Geometry: final body of the model. Coordinates: model frame, mm. A direction names the side the tool comes from. Coordinates: 2 decimals unless noted, no trailing zeros. Loops run counter-clockwise (first coordinate to the right, second up) from the corner with the lowest first, then second, coordinate; pieces in that order, holes last. Notation, with made-up numbers: (41.25, 37) -> (98.25, 37) arc R18 cw to (98.25, 53) -> close; hole circle Ø4 at (-23, 83.25). An arc over 180 degrees is marked (long way). One line per item, written item: value. Start each with the question number.
Item 1: Ray query, probe 1 along Y at (x, z) = (6, 0); probe 2 along Y at (x, z) = (-4, 0); probe 3 along X at (y, z) = (-1.75, -0.25). Return the intervals inside material, ascending. Write a range as from..to.
Item 2: Contact query for flat-ended pins moving along their axis: pin 1 Ø1 at (x, y) = (-7.5, -1) entering from -Z; pin 2 Ø1.5 at (x, y) = (7, 0) entering from +Z; pin 3 Ø4 at (x, y) = (-7, -2.5) entering from +Z. Output: stop coordinate, or through.
Item 3: Section query A-A on y = 0. Return loops of the section in (x, z).
Item 4: Mould query, pull axis X, two halves, no side actions, for faces 1 (the cylindrical face through (5.07, -0.07, -1.5)), 2 (the flat face through (-10, 2, 2)), 3 (the cylindrical face through (-5.81, 0.38, 2.8)), 4 (the cylindrical face through (6.079, 0.845, 2.57)). Classes: +X half, -X half, draft (parallel to the pull), parting line (faces both ways), or undercut.
Item 5: Set-up query: faces 5 (the cylindrical face through (-5, 0, -2)), 6 (the cylindrical face through (-0.136, 3.905, -0.867)). Return all of +Z, -Z, +X, -X, +Y, -Y with unobstructed straight access to the full face (end or side cutting, diameter ignored); none if empty.
Item 6: Section query C-C on x = 5.25. Return loops of the section in (y, z).
Item 7: Section query B-B on z = 0. Return loops of the section in (x, y), then the cut area to 3 significant figures.
Item 8: Section query D-D on z = 3.25. Give the number of separate pieces and of enclosed holes in the cut face, then the cut area to 3 significant figures.
from build123d import *

# Parameters (mm, degrees)
ESQUISSE2_R             = 1.25
ENL_V_MAT_EXTRU_1_DEPTH = 5


with BuildPart() as part:
    # Esquisse1 → Révolution1 (revolve)
    with BuildSketch(Plane.XY, mode=Mode.PRIVATE) as r_volution1_sk:
        Polygon((-10, 3.7), (-10, 2), (0, 2), (0, 1.5), (10, 1.5), (10, 3.7), (9.7, 4), (-9.7, 4), align=None)
    revolve(r_volution1_sk.sketch.rotate(Axis((-9.079951531, 0, 0), (1, 0, 0)), 90), axis=Axis((-9.079951531, 0, 0), (1, 0, 0)))

    # Esquisse2 → Enlèv. mat.-Extru.1 (cut)
    with BuildSketch(Plane.XY.offset(6.1)):
        with Locations((-7, 0)):
            Circle(ESQUISSE2_R)
        with Locations((7, 0)):
            Circle(ESQUISSE2_R)
    extrude(amount=-ENL_V_MAT_EXTRU_1_DEPTH, mode=Mode.SUBTRACT)


solid = part.part
Reply:
1. probe 1: y = -4..-1.5, 1.5..4
1. probe 2: y = -4..-2, 2..4
1. probe 3: x = 0..10
2. pin 1: stops at z = -3.97
2. pin 2: stops at z = -1.3
2. pin 3: stops at z = 3.93
3. outline: (-10, -3.7) -> (-9.7, -4) -> (9.7, -4) -> (10, -3.7) -> (10, -1.5) -> (0, -1.5) -> (0, -2) -> (-10, -2) -> close; (-10, 2) -> (-8.25, 2) -> (-8.25, 4) -> (-9.7, 4) -> (-10, 3.7) -> close; (-5.75, 2) -> (0, 2) -> (0, 1.5) -> (5.75, 1.5) -> (5.75, 4) -> (-5.75, 4) -> close; (8.25, 1.5) -> (10, 1.5) -> (10, 3.7) -> (9.7, 4) -> (8.25, 4) -> close
4. face 1: draft
4. face 2: -X half
4. face 3: undercut
4. face 4: undercut
5. face 5: -X
5. face 6: +X, -X
6. outline: circle Ø8 at (0, 0); hole circle Ø3 at (0, 0)
7. outline: (-10, -3.7) -> (-9.7, -4) -> (9.7, -4) -> (10, -3.7) -> (10, -1.5) -> (0, -1.5) -> (0, -2) -> (-10, -2) -> close; (-10, 2) -> (0, 2) -> (0, 1.5) -> (10, 1.5) -> (10, 3.7) -> (9.7, 4) -> (-9.7, 4) -> (-10, 3.7) -> close
7. area: 89.8 mm²
8. separate pieces: 1
8. enclosed holes: 2
8. area: 83.1 mm²
